Read the model definition and answer for the solid it produces. Units are mm, in the model's axes. Face numbers are marked on the shaded views. A direction names the side the tool comes from. Round coordinates to 2 decimals unless told otherwise and drop trailing zeros. Order: outer loops, then holes, each group sorted by start corner. A loop starts at its lowest first (then second) coordinate and runs counter-clockwise, first axis right, second up.
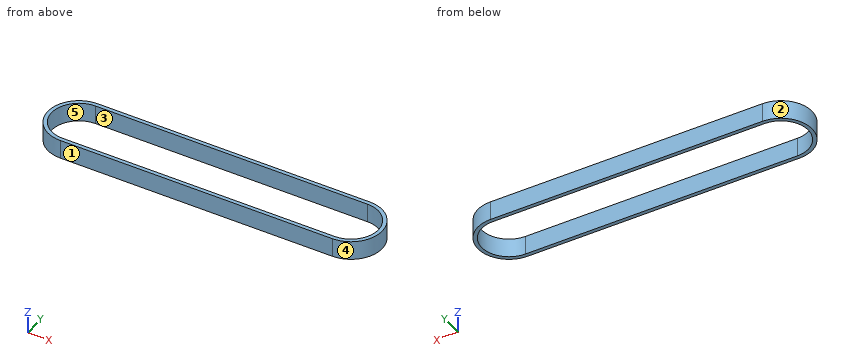
from build123d import *

# Parameters (mm, degrees)
SHEET_EXTRUDE_1_1_DEPTH = 10
THICKEN_1_T1            = 2


with BuildPart() as body_1:
    # Sheet Extrude 1: a surface, the sketch's curves swept straight by 10 mm
    with BuildLine(Plane.XY, mode=Mode.PRIVATE) as sheet_extrude_1_1_path:
        Line((0, -14.435), (-145, -14.435))
        ThreePointArc((-145, -14.435), (-159.435, 0), (-145, 14.435))
        Line((-145, 14.435), (0, 14.435))
        ThreePointArc((0, 14.435), (14.435, 0), (0, -14.435))
    sheet_extrude_1_1 = Shell.extrude(sheet_extrude_1_1_path.wire(), (0 * SHEET_EXTRUDE_1_1_DEPTH, 0 * SHEET_EXTRUDE_1_1_DEPTH, 1 * SHEET_EXTRUDE_1_1_DEPTH))
    add(Solid.thicken(sheet_extrude_1_1, THICKEN_1_T1))


solid = body_1.part
Q1. For the marked faces 4 and 5, determine the directions among +Z, -Z, +X, -X, +Y, -Y from which every point of the face is accessible in a straight line to the end or side of a thin tool.
Outcome:
face 4: +Z, -Z, +X
face 5: +Z, -Z
Q2. For a pull along Y with two mould halves and no side action, classify the marked faces 1, 2 and 3 as released by +Y, released by -Y, zero draft, split by the parting line, or undercut.
Outcome:
face 1: released by -Y
face 2: split by the parting line
face 3: undercut
Q3. A cutting plane is placed at B-B, the plane x = -46. Give the vertices of the cut face in (y, z) (3 decimals).
Outcome:
outline: (-16.435, 0) - (-14.435, 0) - (-14.435, 10) - (-16.435, 10) - close; (14.435, 0) - (16.435, 0) - (16.435, 10) - (14.435, 10) - close
Q4. A cutting plane is placed at C-C, the plane z = 5. Give the vertices of the cut face in (x, y) (3 decimals), plus the area to 3 significant figures.
Outcome:
outline: (-145, -16.435) - (0, -16.435) arc R16.435 ccw to (0, 16.435) - (-145, 16.435) arc R16.435 ccw to start; hole (-145, -14.435) - (0, -14.435) arc R14.435 ccw to (0, 14.435) - (-145, 14.435) arc R14.435 ccw to start
area: 774 mm2
Q5. A cutting plane is placed at A-A, the plane y = 0. Give the vertices of the cut face in (x, z) (3 decimals), plus the area to 3 significant figures.
Outcome:
outline: (-161.435, 0) - (-159.435, 0) - (-159.435, 10) - (-161.435, 10) - close; (14.435, 0) - (16.435, 0) - (16.435, 10) - (14.435, 10) - close
area: 40.0 mm2
Q6. Flat-ended cylindrical pins translate along their axes: pin 1 (5 mm diameter, centred on y = 5, z = 7.5, fed in from -X); pin 2 (5 mm diameter, centred on y = -0.5, z = 1.5, fed in from +X) (3 decimals); pin 3 (5 mm diameter, centred on y = -12, z = 3, fed in from -X); pin 4 (4 mm diameter, centred on y = -11, z = 8, fed in from -X). Find the tip coordinate at first contact, or state that the pin passes through.
Outcome:
pin 1: stops at x = -161.24
pin 2: stops at x = 16.435
pin 3: stops at x = -158.41
pin 4: stops at x = -158.75
Q7. Straight lines are drawn through the part: probe 1 along Y at (x, z) = (-55, 5) (3 decimals); probe 2 along X at (y, z) = (5.5, 8.5); probe 3 along X at (y, z) = (12.5, 1.75). For each, find the intervals that lie inside material, in ascending order.
Outcome:
probe 1: y = -16.435 to -14.435, 14.435 to 16.435
probe 2: x = -160.49 to -158.35, 13.35 to 15.49
probe 3: x = -155.67 to -152.22, 7.22 to 10.67
